Source: three-view drawing plus pictorial views. Frame: mm from the lowest corner of the part. Give positions to 0.01 mm unless a question says otherwise; leave off trailing zeros. Order: outer loops, then holes, each group sorted by start corner. A loop starts at its lowest first (then second) coordinate and runs counter-clockwise, first axis right, second up. Notation, with made-up numbers: (-11.5, 85) - (24.5, 85) arc R23 cw to (24.5, 95) - close; hole circle Ø11 at (12, -0.75). An arc over 180 degrees is marked (long way). Use one line per item in the form item = value.
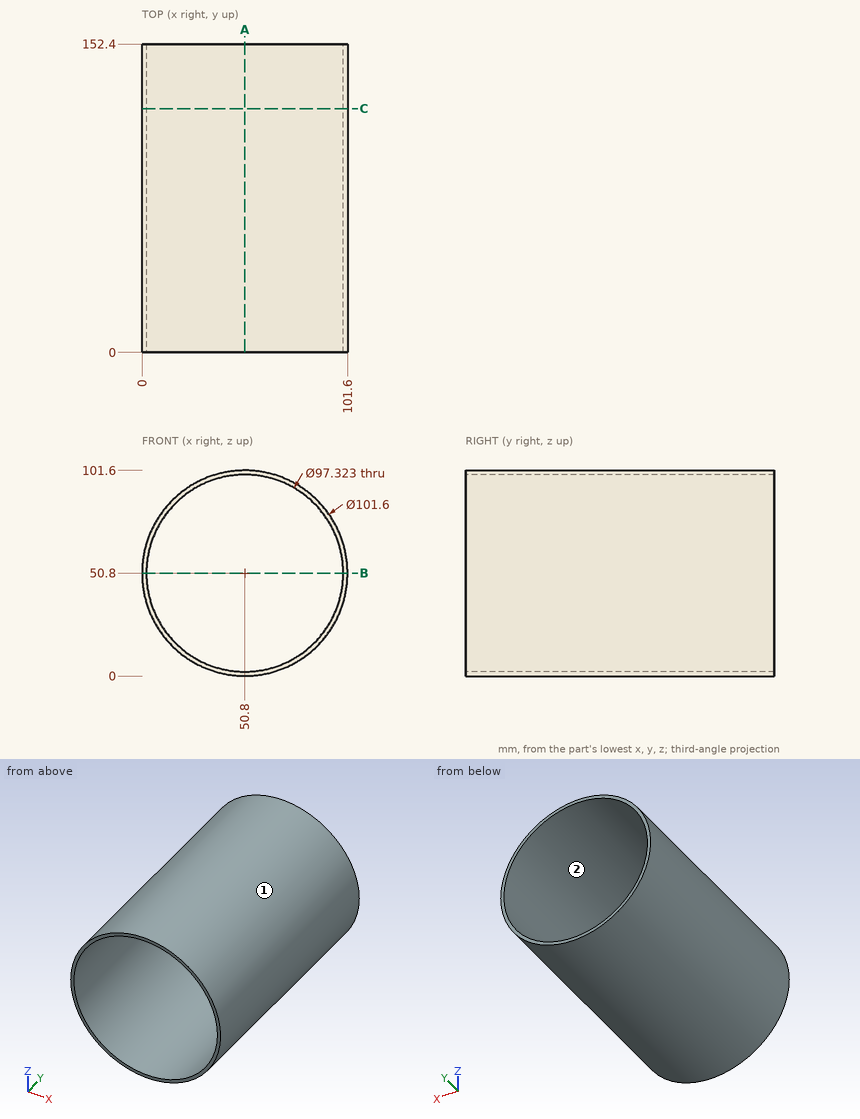
(1) Ray query, line 1 along Z through (x, y) = (50.8, 40); line 2 along X through (y, z) = (52, 50) (1 decimal); line 3 along X through (y, z) = (19, 22.5) (1 decimal). Return the intervals inside material, ascending.
Computed values:
line_1 = 0 to 2.14, 99.46 to 101.6
line_2 = 0 to 2.1, 99.5 to 101.6
line_3 = 8.6 to 11.2, 90.4 to 93
(2) Pull-direction query (X, two-part tool) for the marked faces 1 and 2; classes: released by +X, released by -X, zero draft, split by the parting line, or undercut.
Computed values:
face_1 = split by the parting line
face_2 = undercut
(3) Cut plane A-A on x = 50.8. Output: boundary loops of the cut face in (y, z).
Computed values:
outline = (0, 0) - (152.4, 0) - (152.4, 2.14) - (0, 2.14) - close; (0, 99.46) - (152.4, 99.46) - (152.4, 101.6) - (0, 101.6) - close
(4) Cut plane C-C on y = 120.5. Output: boundary loops of the cut face in (x, z).
Computed values:
outline = circle Ø101.6 at (50.8, 50.8); hole circle Ø97.32 at (50.8, 50.8)
(5) Cut plane B-B on z = 50.8. Output: boundary loops of the cut face in (x, y), plus the area to 3 significant figures.
Computed values:
outline = (0, 0) - (2.14, 0) - (2.14, 152.4) - (0, 152.4) - close; (99.46, 0) - (101.6, 0) - (101.6, 152.4) - (99.46, 152.4) - close
area = 652 mm²
(6) Contact query for flat-ended pins moving along their axis: pin 1 Ø8 at (y, z) = (20, 88.5) entering from -X; pin 2 Ø1.5 at (x, y) = (80, 38) entering from -Z; pin 3 Ø1.5 at (y, z) = (40, 84.5) entering from -X (1 decimal). Output: stop coordinate, or through.
Computed values:
pin_1 = 12.79
pin_2 = 8.71
pin_3 = 12.1
